from build123d import *

# Parameters (mm, degrees)
PAD022_DEPTH             = 10
PAD023_DEPTH             = 20
CLONE091_PITCH_ANGLE     = 90
CLONE091_PLACEMENT_ANGLE = 90
CLONE090_ROLL_ANGLE      = 180
CLONE090_PLACEMENT_ANGLE = -90
CYLINDER1003_R           = 8
CYLINDER1003_DEPTH       = 5
CYLINDER1014_R           = 2.5
CYLINDER1014_DEPTH       = 100
CYLINDER1006_R           = 4
CYLINDER1006_DEPTH       = 70
ARRAY005_Y_COUNT         = 2
ARRAY005_Y_PITCH         = 38
PAD007_DEPTH             = 2.7
ARRAY002_Y_COUNT         = 2
ARRAY002_Y_PITCH         = 20
ARRAY001_Y_COUNT         = 2
ARRAY001_Y_PITCH         = 53
PAD020_DEPTH             = 10
PAD021_DEPTH             = 20
CLONE089_PLACEMENT_ANGLE = 90
ARRAY004_Y_COUNT         = 2
ARRAY004_Y_PITCH         = 20
CLONE088_ROLL_ANGLE      = 180
CLONE088_PLACEMENT_ANGLE = -90
ARRAY003_Y_COUNT         = 2
ARRAY003_Y_PITCH         = 53
PAD_DEPTH                = 20
CHAMFER_1_SIZE           = 16
CHAMFER_2_SIZE           = 5
SKETCH020_W              = 64
SKETCH020_H              = 45
POCKET_DEPTH             = 20.001
SKETCH021_W              = 52.5
SKETCH021_H              = 16
POCKET001_DEPTH          = 20.001
SKETCH022_W              = 25
SKETCH022_H              = 25
PAD019_DEPTH             = 50
CHAMFER017_SIZE          = 5
SKETCH023_W              = 20
SKETCH023_H              = 25
POCKET002_DEPTH          = 50.001
FILLET_1_R               = 4
FILLET_2_R               = 2
EXTRUDE_DEPTH            = 5
ARRAY_Z_COUNT            = 2
ARRAY_Z_PITCH            = 15
SKETCH025_W              = 20
SKETCH025_H              = 60
EXTRUDE001_DEPTH         = 5


with BuildPart() as obj1:
    # Sketch028 → Pad022 (new body)
    with BuildSketch(Plane.XY):
        with BuildLine():
            ThreePointArc((-3.2766, 2.294318), (0, -4), (3.2766, 2.294318))
            Line((0, 6.973787), (3.2766, 2.294318))
            Line((-3.2766, 2.294318), (0, 6.973787))
        make_face()
    extrude(amount=-PAD022_DEPTH)

    # Sketch029 → Pad023 (new body)
    with BuildSketch(Plane.XY):
        with BuildLine():
            ThreePointArc((-1.638314, 1.147138), (0, -2), (1.638314, 1.147138))
            Line((0, 3.486894), (1.638314, 1.147138))
            Line((-1.638314, 1.147138), (0, 3.486894))
        make_face()
    extrude(amount=PAD023_DEPTH)


with BuildPart() as obj2:
    # Clone091 base: copy of obj1
    add(obj1.part)


with BuildPart() as obj2_1:
    # Clone091 pitch: moved
    add(obj2.part.rotate(Axis((0, 0, 0), (0, 1, 0)), CLONE091_PITCH_ANGLE))


with BuildPart() as obj2_2:
    # Clone091 placement: moved
    add(obj2_1.part.moved(Location((-37, -15, 0))).rotate(Axis((-37, -15, 0), (0, 0, 1)), CLONE091_PLACEMENT_ANGLE))


with BuildPart() as obj3:
    # Clone090 base: copy of obj1
    add(obj1.part)


with BuildPart() as obj3_1:
    # Clone090 roll: moved
    add(obj3.part.rotate(Axis((0, 0, 0), (1, 0, 0)), CLONE090_ROLL_ANGLE))


with BuildPart() as obj3_2:
    # Clone090 placement: moved
    add(obj3_1.part.moved(Location((-12, 0, 15))).rotate(Axis((-12, 0, 15), (0, 0, 1)), CLONE090_PLACEMENT_ANGLE))


with BuildPart() as obj4:
    # Cylinder1003 → Cylinder1003 (new body)
    with BuildSketch(Plane.XY):
        Circle(CYLINDER1003_R)
    extrude(amount=CYLINDER1003_DEPTH)


with BuildPart() as obj4_1:
    # Clone093 placement: moved
    add(obj4.part.moved(Location((-10, -42, 5))))


with BuildPart() as obj5:
    # Cylinder1014 → Cylinder1014 (new body)
    with BuildSketch(Plane.XY):
        Circle(CYLINDER1014_R)
    extrude(amount=CYLINDER1014_DEPTH)


with BuildPart() as obj6:
    # Clone095 base: copy of obj5
    add(obj5.part)


with BuildPart() as obj6_1:
    # Clone095 placement: moved
    add(obj6.part.moved(Location((-10, -18.5, 66))))


with BuildPart() as obj7:
    # Clone094 base: copy of obj5
    add(obj5.part)


with BuildPart() as obj7_1:
    # Clone094 placement: moved
    add(obj7.part.moved(Location((-10, -42, 3.5))))


with BuildPart() as obj8:
    # Cylinder1006 → Cylinder1006 (new body)
    with BuildSketch(Plane.XY):
        Circle(CYLINDER1006_R)
    extrude(amount=CYLINDER1006_DEPTH)


with BuildPart() as obj8_1:
    # Clone092 placement: moved
    add(obj8.part.moved(Location((-10, -23, -5))))

    # Array005 Y: obj8_2


with BuildPart() as obj8_2:
    add(obj8_1.part)
    with Locations(*[(0, -i * ARRAY005_Y_PITCH, 0) for i in range(1, ARRAY005_Y_COUNT)]):
        add(obj8_1.part)


with BuildPart() as m3nuthousingmaster:
    # Sketch008 → Pad007 (new body)
    with BuildSketch(Plane.XY):
        Polygon((0, 0), (1.674316, 2.9), (21.674316, 2.9), (21.674316, -2.9), (1.674316, -2.9), align=None)
    extrude(amount=PAD007_DEPTH)


with BuildPart() as lowernuts:
    # Clone087 base: copy of M3NutHousingMaster
    add(m3nuthousingmaster.part)


with BuildPart() as lowernuts_1:
    # Clone087 placement: moved
    add(lowernuts.part.moved(Location((-15, -32, -8))))

    # Array002 Y: LowerNuts ×2


with BuildPart() as lowernuts_2:
    add(lowernuts_1.part)
    with Locations(*[(0, -i * ARRAY002_Y_PITCH, 0) for i in range(1, ARRAY002_Y_COUNT)]):
        add(lowernuts_1.part)


with BuildPart() as lowernuts_3:
    # Array002 placement: moved
    add(lowernuts_2.part.moved(Location((0, 0, 6))))


with BuildPart() as uppernuts:
    # Clone086 base: copy of M3NutHousingMaster
    add(m3nuthousingmaster.part)


with BuildPart() as uppernuts_1:
    # Clone086 placement: moved
    add(uppernuts.part.moved(Location((-14, -15.5, 3.5))))

    # Array001 Y: UpperNuts ×2


with BuildPart() as uppernuts_2:
    add(uppernuts_1.part)
    with Locations(*[(0, -i * ARRAY001_Y_PITCH, 0) for i in range(1, ARRAY001_Y_COUNT)]):
        add(uppernuts_1.part)


with BuildPart() as obj9:
    # Sketch026 → Pad020 (new body)
    with BuildSketch(Plane.XY):
        with BuildLine():
            ThreePointArc((-2.457464, 1.720718), (0, -3), (2.457464, 1.720718))
            Line((0, 5.23034), (2.457464, 1.720718))
            Line((-2.457464, 1.720718), (0, 5.23034))
        make_face()
    extrude(amount=-PAD020_DEPTH)

    # Sketch027 → Pad021 (new body)
    with BuildSketch(Plane.XY):
        with BuildLine():
            ThreePointArc((-1.228737, 0.860352), (0, -1.5), (1.228737, 0.860352))
            Line((0, 2.61517), (1.228737, 0.860352))
            Line((-1.228737, 0.860352), (0, 2.61517))
        make_face()
    extrude(amount=PAD021_DEPTH)


with BuildPart() as lowerbolts:
    # Clone089 base: copy of obj9
    add(obj9.part)


with BuildPart() as lowerbolts_1:
    # Clone089 placement: moved
    add(lowerbolts.part.moved(Location((-10.2, -32, -17))).rotate(Axis((-10.2, -32, -17), (0, 0, 1)), CLONE089_PLACEMENT_ANGLE))

    # Array004 Y: LowerBolts ×2


with BuildPart() as lowerbolts_2:
    add(lowerbolts_1.part)
    with Locations(*[(0, -i * ARRAY004_Y_PITCH, 0) for i in range(1, ARRAY004_Y_COUNT)]):
        add(lowerbolts_1.part)


with BuildPart() as upperbolts:
    # Clone088 base: copy of obj9
    add(obj9.part)


with BuildPart() as upperbolts_1:
    # Clone088 roll: moved
    add(upperbolts.part.rotate(Axis((0, 0, 0), (1, 0, 0)), CLONE088_ROLL_ANGLE))


with BuildPart() as upperbolts_2:
    # Clone088 placement: moved
    add(upperbolts_1.part.moved(Location((-10, -15.5, 12))).rotate(Axis((-10, -15.5, 12), (0, 0, 1)), CLONE088_PLACEMENT_ANGLE))

    # Array003 Y: UpperBolts ×2


with BuildPart() as upperbolts_3:
    add(upperbolts_2.part)
    with Locations(*[(0, -i * ARRAY003_Y_PITCH, 0) for i in range(1, ARRAY003_Y_COUNT)]):
        add(upperbolts_2.part)


with BuildPart() as obj10:
    # Sketch → Pad (new body)
    with BuildSketch(Plane.YZ):
        Polygon((0, 86), (-79, 86), (-79, -10), (-5, -10), (-5, 52.339746), (0, 61), align=None)
    extrude(amount=-PAD_DEPTH)

    # Chamfer 1
    chamfer_1_edges = [obj10.edges().sort_by_distance(p)[0] for p in [
        (-10, -79, 86),
    ]]
    chamfer(chamfer_1_edges, length=CHAMFER_1_SIZE)

    # Chamfer 2
    chamfer_2_edges = [obj10.edges().sort_by_distance(p)[0] for p in [
        (-10, 0, 86),
    ]]
    chamfer(chamfer_2_edges, length=CHAMFER_2_SIZE)

    # Sketch020 → Pocket (cut, through all)
    with BuildSketch(Plane.YZ):
        with Locations((-42, 37.5)):
            Rectangle(SKETCH020_W, SKETCH020_H)
    extrude(amount=-POCKET_DEPTH, mode=Mode.SUBTRACT)

    # Sketch021 → Pocket001 (cut, through all)
    with BuildSketch(Plane.YZ):
        with Locations((-33.75, 75.5)):
            Rectangle(SKETCH021_W, SKETCH021_H)
    extrude(amount=-POCKET001_DEPTH, mode=Mode.SUBTRACT)

    # Sketch022 → Pad019 (new body)
    with BuildSketch(Plane.YZ):
        with Locations((-2.5, 2.5)):
            Rectangle(SKETCH022_W, SKETCH022_H)
    extrude(amount=-PAD019_DEPTH)

    # Chamfer017
    chamfer017_edges = [obj10.edges().sort_by_distance(p)[0] for p in [
        (-10, -5, 15),
    ]]
    chamfer(chamfer017_edges, length=CHAMFER017_SIZE)

    # Sketch023 → Pocket002 (cut, through all)
    with BuildSketch(Plane.YZ):
        with Locations((0, -2.5)):
            Rectangle(SKETCH023_W, SKETCH023_H)
    extrude(amount=-POCKET002_DEPTH, mode=Mode.SUBTRACT)

    # Fillet 1
    fillet_1_edges = [obj10.edges().sort_by_distance(p)[0] for p in [
        (-35, -15, 15),
    ]]
    fillet(fillet_1_edges, radius=FILLET_1_R)

    # Fillet 2
    fillet_2_edges = [obj10.edges().sort_by_distance(p)[0] for p in [
        (-10, -5, 20),
        (-10, -5, 52.339746),
        (-10, 0, 15),
        (-10, 0, 61),
        (-10, 0, 81),
        (-10, -5, 86),
        (-10, -63, 86),
        (-10, -79, 70),
    ]]
    fillet(fillet_2_edges, radius=FILLET_2_R)


with BuildPart() as componentscut:
    # Sketch024 → Extrude (new body)
    with BuildSketch(Plane.XY.offset(15)):
        with BuildLine():
            Line((-42, -12), (-18, -12))
            Line((-18, -12), (-18, -67))
            add(Edge.make_bspline(
                [(-18, -67), (-21.374537, -28.653178), (-42, -12)],
                knots=[4.860682, 4.860682, 4.860682, 5.839233, 5.839233, 5.839233], degree=2, weights=[1, 0.882673, 1]))
        make_face()
    extrude(amount=-EXTRUDE_DEPTH)


with BuildPart() as componentscut_1:
    # Extrude placement: moved
    add(componentscut.part.moved(Location((0, 0, -5))))

    # Array Z: ComponentsCut ×2


with BuildPart() as componentscut_2:
    add(componentscut_1.part)
    with Locations(*[(0, 0, -i * ARRAY_Z_PITCH) for i in range(1, ARRAY_Z_COUNT)]):
        add(componentscut_1.part)

    # Fusion: union obj10
    add(obj10.part)

    # Cut: cut UpperBolts
    add(upperbolts_3.part, mode=Mode.SUBTRACT)

    # Cut001: cut LowerBolts
    add(lowerbolts_2.part, mode=Mode.SUBTRACT)

    # Cut002: cut UpperNuts
    add(uppernuts_2.part, mode=Mode.SUBTRACT)

    # Cut003: cut LowerNuts
    add(lowernuts_3.part, mode=Mode.SUBTRACT)

    # Cut004: cut obj8
    add(obj8_2.part, mode=Mode.SUBTRACT)

    # Cut005: cut obj7
    add(obj7_1.part, mode=Mode.SUBTRACT)

    # Cut006: cut obj6
    add(obj6_1.part, mode=Mode.SUBTRACT)

    # Cut007: cut obj4
    add(obj4_1.part, mode=Mode.SUBTRACT)

    # Cut008: cut obj3
    add(obj3_2.part, mode=Mode.SUBTRACT)

    # Cut009: cut obj2
    add(obj2_2.part, mode=Mode.SUBTRACT)


with BuildPart() as upperlidcommon:
    # Sketch025 → Extrude001 (new body)
    with BuildSketch(Plane.XY.offset(15)):
        with Locations((-10, -42)):
            Rectangle(SKETCH025_W, SKETCH025_H)
    extrude(amount=-EXTRUDE001_DEPTH)

    # Common: intersect ComponentsCut
    add(componentscut_2.part, mode=Mode.INTERSECT)


solid = upperlidcommon.part
For this review, take the finished solid that the model builds, in its own axes (mm). A direction names the side the tool comes from. Coordinates: 2 decimals unless noted, no trailing zeros. Loops run counter-clockwise (first coordinate to the right, second up) from the corner with the lowest first, then second, coordinate; pieces in that order, holes last. Notation, with made-up numbers: (-30.75, 66.5) -> (-0.75, 66.5) arc R10 ccw to (-0.75, 72.5) -> close; hole circle Ø8 at (-29.5, -30.5). An arc over 180 degrees is marked (long way). Write each question's results on one line, items separated by ' | '.
Q1. Add section C-C, the plane z = 13.4. State the section outline as (x, y) points, then the cut area to 3 significant figures.
Taken from the geometry:
outline: (-20, -72) -> (0, -72) -> (0, -12) -> (-20, -12) -> close; hole (-15.23, -68.5) -> (-11.72, -70.96) arc R3 ccw (long way) to (-11.72, -66.04) -> close; hole (-15.23, -15.5) -> (-11.72, -17.96) arc R3 ccw (long way) to (-11.72, -13.04) -> close; hole circle Ø8 at (-10, -61); hole circle Ø8 at (-10, -23); hole circle Ø5 at (-10, -42) | area: 1,010 mm²
Q2. To check wall thickness, follow line 1 along Y through (x, z) = (-10, 10.55); line 2 along Y through (x, z) = (-10, 13.9); line 3 along X through (y, z) = (-61, 12.5). State the ranges of each line that lie inside material, in increasing order. Write a range as [from, to].
Taken from the geometry:
line 1: [-72, -70], [-67, -65], [-57, -44.5], [-39.5, -27], [-19, -17], [-14, -12] | line 2: [-72, -71.5], [-65.5, -65], [-57, -44.5], [-39.5, -27], [-19, -18.5], [-12.5, -12] | line 3: [-20, -14], [-6, 0]
Q3. For pin 1 Ø5.5 at (x, y) = (-10, -68.5) entering from +Z; pin 2 Ø4 at (x, y) = (-10, -42) entering from +Z, all flat-tipped, find the tip position at first contact; note any pin that passes through.
Taken from the geometry:
pin 1: z = 12 | pin 2: through
Q4. Add section B-B, the plane y = -23. State the section outline as (x, z) points, then the cut area to 3 significant figures.
Taken from the geometry:
outline: (-20, 10) -> (-14, 10) -> (-14, 15) -> (-20, 15) -> close; (-6, 10) -> (0, 10) -> (0, 15) -> (-6, 15) -> close | area: 60.0 mm²
Q5. Mouldability with a two-part tool opening along X and no side actions: class faces 4 (the flat face through (0, -42, 13)), 5 (the flat face through (-6, -42, 15)), 6 (the cylindrical face through (-8.5, -68.5, 11)) as +X half, -X half, draft (parallel to the pull), parting line (faces both ways), or undercut.
Taken from the geometry:
face 4: +X half | face 5: draft | face 6: undercut
Q6. Add section D-D, the plane z = 10.8. State the section outline as (x, y) points.
Taken from the geometry:
outline: (-20, -72) -> (0, -72) -> (0, -12) -> (-20, -12) -> close; hole circle Ø8 at (-10, -61); hole circle Ø8 at (-10, -23); hole (-12.62, -68.5) -> (-10.86, -69.73) arc R1.5 ccw (long way) to (-10.86, -67.27) -> close; hole (-12.62, -15.5) -> (-10.86, -16.73) arc R1.5 ccw (long way) to (-10.86, -14.27) -> close; hole circle Ø5 at (-10, -42)
Q7. Add section A-A, the plane x = -10. Count the separate pieces of the cut face and the enclosed holes in it, then the cut area to 3 significant figures.
Taken from the geometry:
separate pieces: 6 | enclosed holes: 0 | area: 147 mm²
Q8. Machinability: for faces 1 (the flat face through (-13.451, -67.254, 13.479)), 2 (the flat face through (-10, -72, 13)), 3 (the flat face through (-11.75, -16.106, 11.014)), which of the approach directions +Z, -Z, +X, -X, +Y, -Y give a long, thin tool a straight path to every point of the face, cutting with its end or side? Answer none if there is none.
Taken from the geometry:
face 1: +Z | face 2: +Z, -Z, +X, -X, -Y | face 3: +Z, -Z
